Work out the finished part from the listing and answer in its coordinate system (mm). Round coordinates to 2 decimals unless told otherwise and drop trailing zeros. Loops run counter-clockwise (first coordinate to the right, second up) from the corner with the lowest first, then second, coordinate; pieces in that order, holes last.
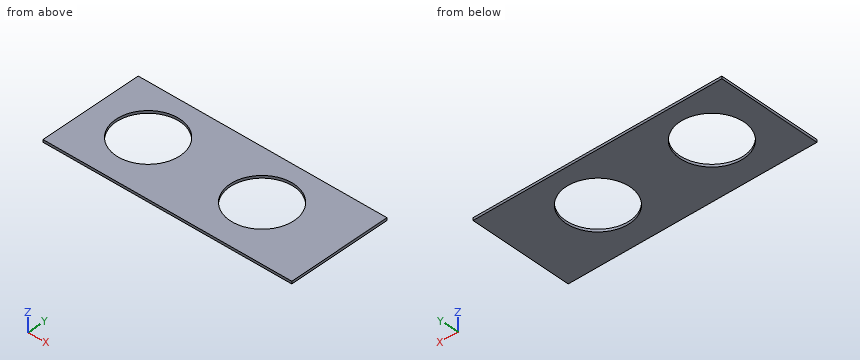
```python
from build123d import *

# Parameters (mm, degrees)
F1_W     = 310.345411
F1_H     = 128.536235
F1_R     = 40
F3_DEPTH = 3.175
F4_R     = 40
F5_DEPTH = 25.4


with BuildPart() as f3:
    # F1 (on face) → F3 (new body)
    with BuildSketch(Plane.XY):
        with Locations((6.08109, 46.009373)):
            Rectangle(F1_W, F1_H)
        with Locations((-80.468008, 49.394639)):
            Circle(F1_R, mode=Mode.SUBTRACT)
    extrude(amount=F3_DEPTH)

    # F4 (on face) → F5 (cut)
    with BuildSketch(Plane.XY):
        with Locations((61.672111, 49.394639)):
            Circle(F4_R)
    extrude(amount=F5_DEPTH, mode=Mode.SUBTRACT)


solid = f3.part
```
1. Find section A-A (x = 30). Write down the section's boundary in (y, z) (1 decimal).
Answer key:
outline: (-18.3, 0) - (25, 0) - (25, 3.2) - (-18.3, 3.2) - close; (73.8, 0) - (110.3, 0) - (110.3, 3.2) - (73.8, 3.2) - close
2. Find section C-C (x = -102.5). Write down the section's boundary in (y, z) (1 decimal).
Answer key:
outline: (-18.3, 0) - (16, 0) - (16, 3.2) - (-18.3, 3.2) - close; (82.8, 0) - (110.3, 0) - (110.3, 3.2) - (82.8, 3.2) - close
3. Find section D-D (z = 0.75). Write down the section's boundary in (x, y), then the cut area to 3 significant figures.
Answer key:
outline: (-149.09, -18.26) - (161.25, -18.26) - (161.25, 110.28) - (-149.09, 110.28) - close; hole circle Ø80 at (-80.47, 49.39); hole circle Ø80 at (61.67, 49.39)
area: 29,800 mm2
4. Consider probe 1 along X at (y, z) = (49, 2.85); probe 2 along X at (y, z) = (39.5, 0.35); probe 3 along Y at (x, z) = (-80, 2.5). Determine where each line is inside the solid, lowest interval first.
Answer key:
probe 1: x = -149.09 to -120.47, -40.47 to 21.67, 101.67 to 161.25
probe 2: x = -149.09 to -119.22, -41.71 to 22.92, 100.43 to 161.25
probe 3: y = -18.26 to 9.4, 89.39 to 110.28
5. Find section B-B (y = 44). Write down the section's boundary in (x, z) (3 decimals), then the cut area to 3 significant figures.
Answer key:
outline: (-149.092, 0) - (-120.103, 0) - (-120.103, 3.175) - (-149.092, 3.175) - close; (-40.833, 0) - (22.038, 0) - (22.038, 3.175) - (-40.833, 3.175) - close; (101.307, 0) - (161.254, 0) - (161.254, 3.175) - (101.307, 3.175) - close
area: 482 mm2
